```python
from build123d import *

# Parameters (mm, degrees)
SKETCH1_W           = 100
SKETCH1_H           = 150
BOSS_EXTRUDE1_DEPTH = 5
SKETCH2_W           = 2.543215169
SKETCH2_H           = 18.583792384
BOSS_EXTRUDE2_DEPTH = 5


with BuildPart() as part:
    # Sketch1 → Boss-Extrude1 (new body)
    with BuildSketch(Plane.XY):
        Rectangle(SKETCH1_W, SKETCH1_H)
    extrude(amount=BOSS_EXTRUDE1_DEPTH)

    # Sketch2 → Boss-Extrude2 (add)
    with BuildSketch(Plane.XY.offset(5)):
        with Locations((-35.723415387, 0)):
            Rectangle(SKETCH2_W, SKETCH2_H)
    boss_extrude2 = extrude(amount=BOSS_EXTRUDE2_DEPTH)

    # Mirror1: Boss-Extrude2 across plane
    add(boss_extrude2.mirror(Plane(origin=(0, 0, 0), x_dir=(0, 0, 1), z_dir=(1, 0, 0))))


solid = part.part
```
Work out the finished part from the listing and answer in its coordinate system (mm). A direction names the side the tool comes from. Give positions to 0.01 mm unless a question says otherwise; leave off trailing zeros. Write each loop counter-clockwise with the first axis right and the second up, starting at its lowest first coordinate (ties: lowest second). Pieces come first, ordered by that corner, then holes.
(1) Flat-ended cylindrical pins translate along their axes: pin 1 Ø6 at (x, y) = (-16, -10) entering from -Z; pin 2 Ø2.5 at (y, z) = (-0.5, 7) entering from +X (3 decimals); pin 3 Ø1.3 at (x, z) = (-35.5, 8) entering from -Y; pin 4 Ø3 at (x, z) = (-35.5, 8) entering from +Y. Find the tip coordinate at first contact, or state that the pin passes through.
Final values:
pin 1: stops at z = 0
pin 2: stops at x = 36.995
pin 3: stops at y = -9.29
pin 4: stops at y = 9.29
(2) The part is cut by section C-C on x = 16.5. Write down the section's boundary in (y, z).
Final values:
outline: (-75, 0) - (75, 0) - (75, 5) - (-75, 5) - close
(3) Which of the six approach directions +Z, -Z, +X, -X, +Y, -Y give full straight-line access (tool end or side, diameter ignored) to faces 4 (the flat face through (-1, -75, 2)), 5 (the flat face through (-36.995, 0, 7)), 6 (the flat face through (34.452, 0, 7))?
Final values:
face 4: +Z, -Z, +X, -X, -Y
face 5: +Z, -X, +Y, -Y
face 6: +Z, +Y, -Y
(4) The part is cut by section A-A on z = 6.75. Write down the section's boundary in (x, y).
Final values:
outline: (-37, -9.29) - (-34.45, -9.29) - (-34.45, 9.29) - (-37, 9.29) - close; (34.45, -9.29) - (37, -9.29) - (37, 9.29) - (34.45, 9.29) - close
(5) The part is cut by section B-B on y = 42. Write down the section's boundary in (x, z).
Final values:
outline: (-50, 0) - (50, 0) - (50, 5) - (-50, 5) - close
(6) Straight lines are drawn through the part: line 1 (Z direction, x = -10.5, y = -64.5); line 2 (X direction, y = 2.5, z = 9.5). For each, find the intervals that lie inside material, in ascending order.
Final values:
line 1: z = 0 to 5
line 2: x = -37 to -34.45, 34.45 to 37
(7) The mould has two halves that part along X. Classify faces 1 (the flat face through (-34.452, 0, 7)), 2 (the flat face through (36.995, 0, 7)), 3 (the flat face through (-1, 75, 2)): pulls with the +X half, pulls with the -X half, needs draft (parallel to the pull), parting line crosses it, or undercut.
Final values:
face 1: undercut
face 2: pulls with the +X half
face 3: needs draft
